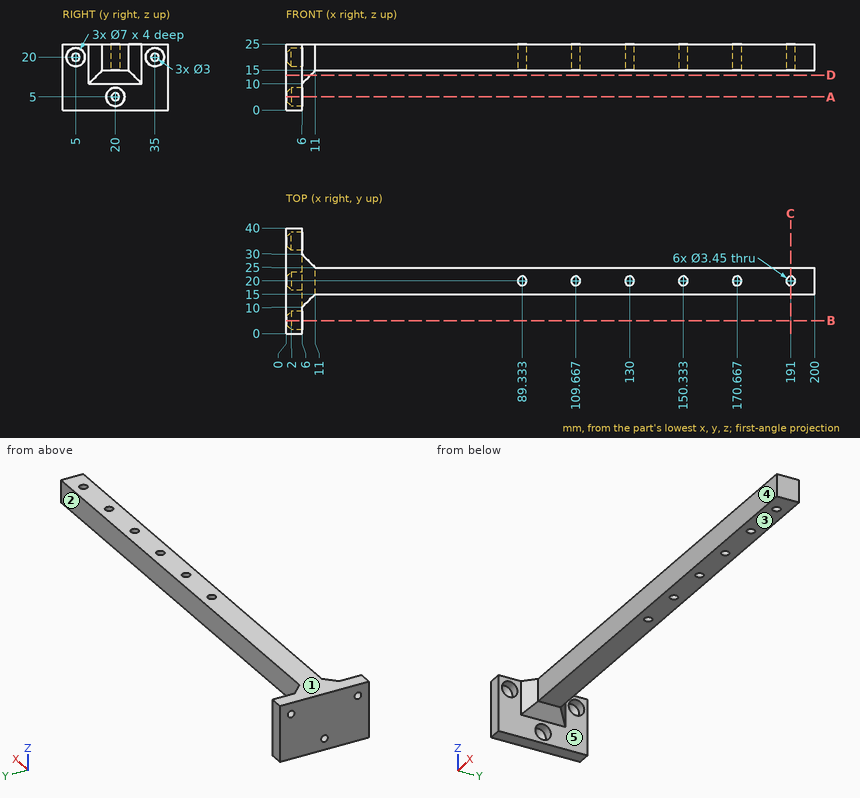
Part print with two shaded views. Sizes in mm from the minimum x, y, z corner. A direction names the side the tool comes from. Give positions to 0.01 mm unless a question says otherwise; leave off trailing zeros. Write each loop counter-clockwise with the first axis right and the second up, starting at its lowest first coordinate (ties: lowest second). Pieces come first, ordered by that corner, then holes.
1) Cut at C-C on x = 191. Write the cut outline in (y, z) (1 decimal).
Resolved:
outline: (15, 15) - (18.3, 15) - (18.3, 25) - (15, 25) - close; (21.7, 15) - (25, 15) - (25, 25) - (21.7, 25) - close
2) Probe L1, parallel to Z at x = 3.05, y = 35; L2, parallel to Y at x = 191, z = 17 (1 decimal); L3, parallel to X at y = 7.5, z = 23.75. List the from-to ranges inside material, lowest first.
Resolved:
L1: z = 0 to 16.5, 23.5 to 25
L2: y = 15 to 18.3, 21.7 to 25
L3: x = 0 to 6
3) Cut at B-B on y = 5. Write the cut outline in (x, z), then the cut area to 3 significant figures.
Resolved:
outline: (0, 0) - (6, 0) - (6, 16.5) - (2, 16.5) - (0, 18.5) - close; (0, 21.5) - (2, 23.5) - (6, 23.5) - (6, 25) - (0, 25) - close
area: 112 mm2
4) Pin check, flat tips, straight feed: pin 1 (8 mm diameter, centred on x = 92.5, z = 19.5, fed in from +Y); pin 2 (11 mm diameter, centred on x = 73.5, y = 18, fed in from -Z); pin 3 (3 mm diameter, centred on x = 115, z = 18.5, fed in from -Y). Stop position of each tip, or through.
Resolved:
pin 1: stops at y = 25
pin 2: stops at z = 15
pin 3: stops at y = 15
5) Cut at D-D on z = 13.25. Write the cut outline in (x, y).
Resolved:
outline: (0, 0) - (6, 0) - (6, 10) - (9.25, 13.25) - (9.25, 26.75) - (6, 30) - (6, 40) - (0, 40) - close
6) Cut at A-A on z = 5. Write the cut outline in (x, y), then the cut area to 3 significant figures.
Resolved:
outline: (0, 0) - (6, 0) - (6, 16.5) - (2, 16.5) - (0, 18.5) - close; (0, 21.5) - (2, 23.5) - (6, 23.5) - (6, 40) - (0, 40) - close
area: 202 mm2
7) Which spindle directions (+Z, -Z, +X, -X, +Y, -Y) get a long thin tool onto all of the face, cutting with end or side? Do the marked faces 1, 2, 3, 4 and 5. Say none if no direction does.
Resolved:
face 1: +Z, +X, -X, +Y, -Y
face 2: +Z, -Z, +X, +Y
face 3: -Z, +X, +Y, -Y
face 4: +Z, -Z, +X, -Y
face 5: -Z, +X
